Here's how the part is built. I have some questions about the finished solid (model axes, mm). Give positions to 0.01 mm unless a question says otherwise; leave off trailing zeros. Loops run counter-clockwise (first coordinate to the right, second up) from the corner with the lowest first, then second, coordinate; pieces in that order, holes last.
Q1. If we section it at A-A (y = 154.5): Please give me the cut outline in (x, z), plus the area to 3 significant figures.
Q2. I need wall thicknesses on line 1 (X direction, y = 164, z = 2.25); line 2 (Y direction, x = -4.67, z = 1.7); line 3 (X direction, y = 64, z = 3.1). Which ranges of each line are inside material? Lowest first, please.
Q3. If we section it at B-B (z = 1.85): Give the number of separate pieces and of enclosed holes in the cut face, plus the area to 3 significant figures.
from build123d import *

# Parameters (mm, degrees)
SKETCH1_R           = 5
BOSS_EXTRUDE1_DEPTH = 5
SKETCH4_W           = 4
SKETCH4_H           = 60
CUT_EXTRUDE1_DEPTH  = 10
SKETCH5_R           = 1.5
SKETCH5_W           = 6
SKETCH5_H           = 27.65
CUT_EXTRUDE2_DEPTH  = 6
FILLET1_R           = 10


with BuildPart() as part:
    # Sketch1 → Boss-Extrude1 (new body)
    with BuildSketch(Plane.XY):
        Polygon((100, 190), (-100, 190), (-100, -90), (-100, -160), (100, -160), (100, -90), align=None)
        with Locations((-57.587555345, 115.778221854)):
            Circle(SKETCH1_R, mode=Mode.SUBTRACT)
        with Locations((57.587555345, 115.778221854)):
            Circle(SKETCH1_R, mode=Mode.SUBTRACT)
        with Locations((57.587555345, -85.778221854)):
            Circle(SKETCH1_R, mode=Mode.SUBTRACT)
        with Locations((-57.587555345, -85.778221854)):
            Circle(SKETCH1_R, mode=Mode.SUBTRACT)
    extrude(amount=BOSS_EXTRUDE1_DEPTH)

    # Sketch4 → Cut-Extrude1 (cut)
    with BuildSketch(Plane.XY.offset(5)):
        Polygon((1, 73), (1, 58), (5, 58), (5, 118), (1, 118), (1, 103), (-9, 103), (-9, 73), align=None)
        with Locations((47, 88)):
            Rectangle(SKETCH4_W, SKETCH4_H)
    extrude(amount=-CUT_EXTRUDE1_DEPTH, mode=Mode.SUBTRACT)

    # Sketch5 → Cut-Extrude2 (cut, through all)
    with BuildSketch(Plane.XY.offset(5)):
        with Locations((4.67, -155)):
            Circle(SKETCH5_R)
        with Locations((-4.67, -155)):
            Circle(SKETCH5_R)
        with Locations((-87, 152.175)):
            Rectangle(SKETCH5_W, SKETCH5_H)
        with Locations((-87, 111.115)):
            Rectangle(SKETCH5_W, SKETCH5_H)
        with Locations((-87, -87.845)):
            Rectangle(SKETCH5_W, SKETCH5_H)
        with Locations((-87, -128.905)):
            Rectangle(SKETCH5_W, SKETCH5_H)
        with Locations((87, -87.845)):
            Rectangle(SKETCH5_W, SKETCH5_H)
        with Locations((87, -128.905)):
            Rectangle(SKETCH5_W, SKETCH5_H)
        with Locations((87, 152.175)):
            Rectangle(SKETCH5_W, SKETCH5_H)
        with Locations((87, 111.115)):
            Rectangle(SKETCH5_W, SKETCH5_H)
    extrude(amount=-CUT_EXTRUDE2_DEPTH, mode=Mode.SUBTRACT)

    # Fillet1
    fillet1_edges = [part.edges().sort_by_distance(p)[0] for p in [
        (-100, 190, 2.5),
        (100, 190, 2.5),
        (100, -160, 2.5),
        (-100, -160, 2.5),
    ]]
    fillet(fillet1_edges, radius=FILLET1_R)


solid = part.part
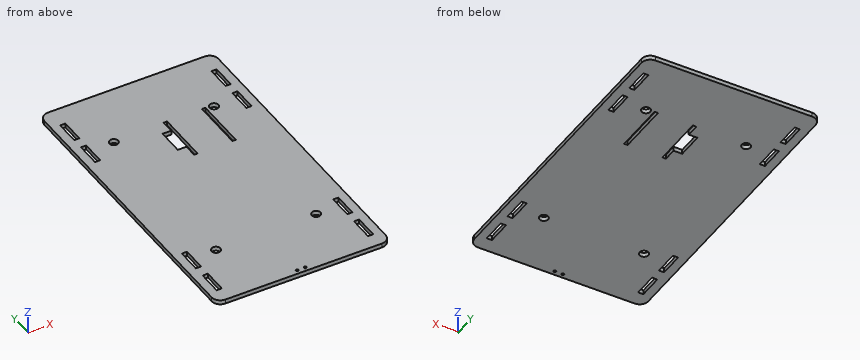
Check sheet entries:
1. outline: (-100, 0) - (-90, 0) - (-90, 5) - (-100, 5) - close; (-84, 0) - (84, 0) - (84, 5) - (-84, 5) - close; (90, 0) - (100, 0) - (100, 5) - (90, 5) - close
1. area: 940 mm2
2. line 1: x = -100 to -90, -84 to 84, 90 to 100
2. line 2: y = -160 to -156.5, -153.5 to 73, 103 to 190
2. line 3: x = -100 to 1, 5 to 45, 49 to 100
3. separate pieces: 1
3. enclosed holes: 16
3. area: 67,500 mm2
